Geometry: see drawing. Coordinates: mm, zero at the bounding-box minimum. A direction names the side the tool comes from. Round coordinates to 2 decimals unless told otherwise and drop trailing zeros. Loops run counter-clockwise (first coordinate to the right, second up) from the corner with the lowest first, then second, coordinate; pieces in that order, holes last.
(1) Mould query, pull axis X, two halves, no side actions, for the marked faces 1, 2 and 3. Classes: pulls with the +X half, pulls with the -X half, needs draft (parallel to the pull), parting line crosses it, or undercut.
(2) First-contact query: pin 1 Ø1 at (x, y) = (37.5, 8.5) entering from +Z. Flat tip, straight axial feed; report the tip coordinate or a pass-through.
(3) Section A-A, the plane x = 26. Return the cut outline in (y, z).
(4) Set-up query: the marked faces 4 and 5. Return all of +Z, -Z, +X, -X, +Y, -Y with unobstructed straight access to the full face (end or side cutting, diameter ignored); none if empty.
(5) Section B-B, the plane y = 6.5. Return the cut outline in (x, z), plus the area to 3 significant figures.
(6) Section C-C, the plane z = 18. Return the cut outline in (x, y).
(7) Material intervals for probe 1 along X at (y, z) = (11, 22.5); probe 2 along Y at (x, z) = (26, 1.7); probe 3 along Z at (x, y) = (21, 4.5), sorted ascending.
(8) Section D-D, the plane y = 9.25. Return the cut outline in (x, z), plus the area to 3 significant figures.
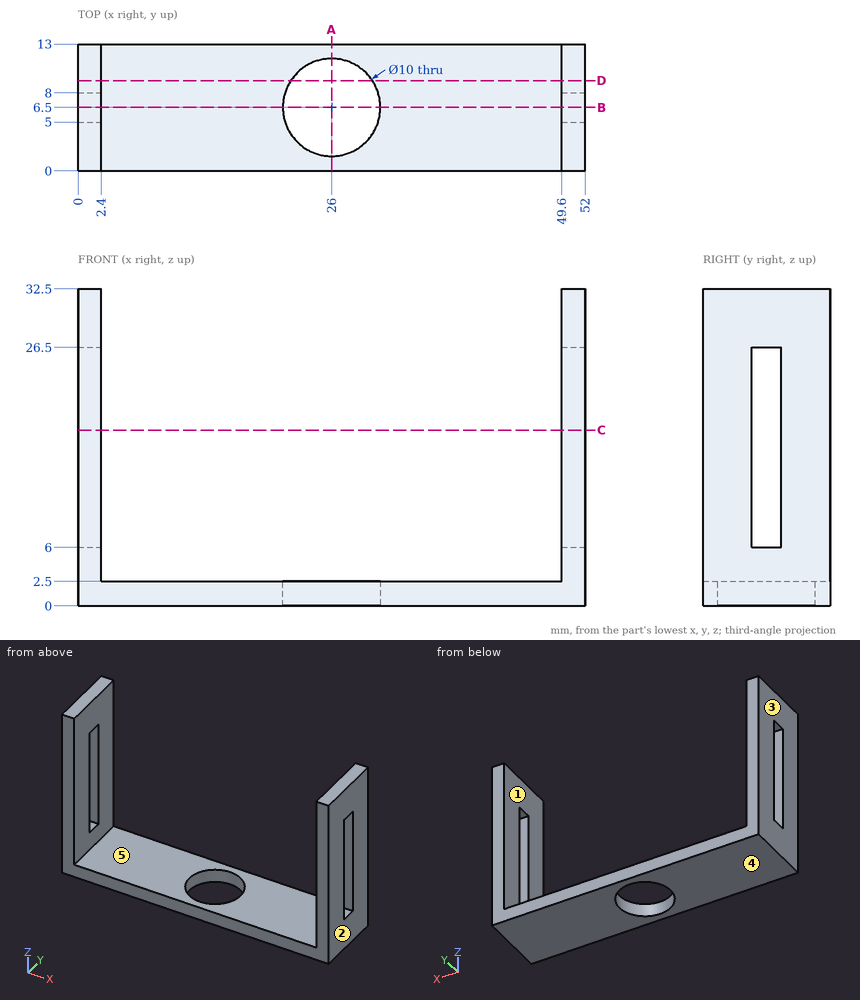
Output values:
1. face 1: undercut
1. face 2: pulls with the +X half
1. face 3: pulls with the -X half
2. pin 1: stops at z = 2.5
3. outline: (0, 0) - (1.5, 0) - (1.5, 2.5) - (0, 2.5) - close; (11.5, 0) - (13, 0) - (13, 2.5) - (11.5, 2.5) - close
4. face 4: -Z, +X, -X, +Y, -Y
4. face 5: +Z, +Y, -Y
5. outline: (0, 0) - (21, 0) - (21, 2.5) - (2.4, 2.5) - (2.4, 6) - (0, 6) - close; (0, 26.5) - (2.4, 26.5) - (2.4, 32.5) - (0, 32.5) - close; (31, 0) - (52, 0) - (52, 6) - (49.6, 6) - (49.6, 2.5) - (31, 2.5) - close; (49.6, 26.5) - (52, 26.5) - (52, 32.5) - (49.6, 32.5) - close
5. area: 151 mm2
6. outline: (0, 0) - (2.4, 0) - (2.4, 5) - (0, 5) - close; (0, 8) - (2.4, 8) - (2.4, 13) - (0, 13) - close; (49.6, 0) - (52, 0) - (52, 5) - (49.6, 5) - close; (49.6, 8) - (52, 8) - (52, 13) - (49.6, 13) - close
7. probe 1: x = 0 to 2.4, 49.6 to 52
7. probe 2: y = 0 to 1.5, 11.5 to 13
7. probe 3: z = 0 to 2.5
8. outline: (0, 0) - (21.82, 0) - (21.82, 2.5) - (2.4, 2.5) - (2.4, 32.5) - (0, 32.5) - close; (30.18, 0) - (52, 0) - (52, 32.5) - (49.6, 32.5) - (49.6, 2.5) - (30.18, 2.5) - close
8. area: 253 mm2
